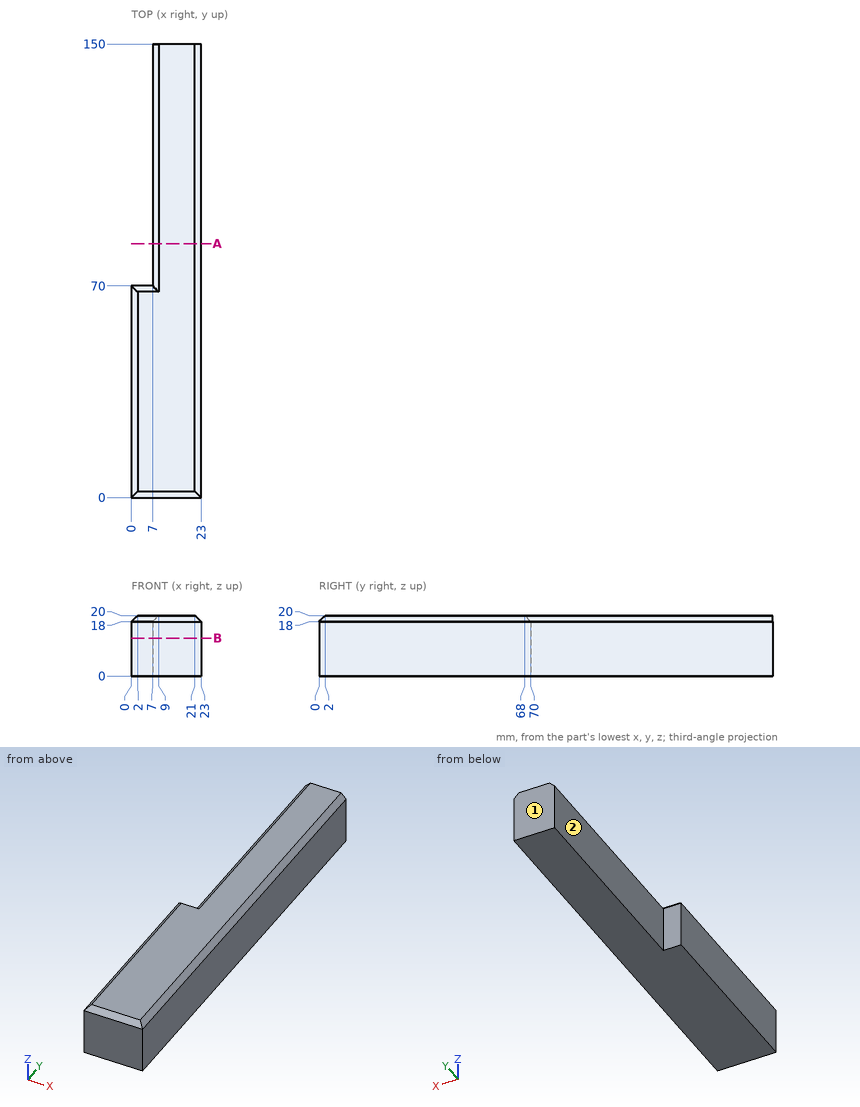
Verification items for this drawing (mm, ordinates from the low corner). A direction names the side the tool comes from. Coordinates: 2 decimals unless noted, no trailing zeros. Write each loop counter-clockwise with the first axis right and the second up, starting at its lowest first coordinate (ties: lowest second). Pieces come first, ordered by that corner, then holes. Notation, with made-up numbers: M 76,9 L 96,9 A31 ccw 96,42 Z; hole C 8.5,-2.75 d6. An arc over 180 degrees is marked long. Answer as a JSON object with one key per item and string values. Group by question number.
(1) Gauge pin test, flat ends, axial feed: pin 1 (5.5 mm diameter, centred on y = 98.5, z = 10.5, fed in from -X); pin 2 (7.5 mm diameter, centred on x = 3.5, z = 7, fed in from +Y); pin 3 (1.5 mm diameter, centred on x = 7.5, y = 133, fed in from +Z). Record the tip position at first contact, or that the pin passes through.
(2) Material ranges on line 1 (X direction, y = 81.5, z = 14); line 2 (Y direction, x = 3.75, z = 14.5); line 3 (X direction, y = 64, z = 18.5), recorded low to high.
(3) Cross-section at B-B, the plane z = 12.5. Record the cut outline in (x, y), and give its area (3 significant figures).
(4) Cross-section at A-A, the plane y = 84. Record the cut outline in (x, z), and give its area (3 significant figures).
(5) Tool access check on the marked faces 1 and 2. Record the directions out of +Z, -Z, +X, -X, +Y, -Y that give a thin tool (end or side, any length) a straight path to the whole face; none if there is none.
Reply:
{
 "1": {"pin 1": "x = 7", "pin 2": "y = 150", "pin 3": "z = 19.25"},
 "2": {"line 1": "7 to 23", "line 2": "0 to 70", "line 3": "0.5 to 22.5"},
 "3": {"outline": "M 0,0 L 23,0 L 23,150 L 7,150 L 7,70 L 0,70 Z", "area": "2,890 mm²"},
 "4": {"outline": "M 7,0 L 23,0 L 23,18 L 21,20 L 9,20 L 7,18 Z", "area": "316 mm²"},
 "5": {"face 1": "+Z, -Z, +X, -X, +Y", "face 2": "+Z, -Z, -X, +Y"}
}
